Autodesk Inventor part; units mm, degrees
ref_plane "YZ Plane" through (0, 0, 0) normal (1, 0, 0) x (0, 1, 0)
ref_plane "XZ Plane" through (0, 0, 0) normal (0, 1, 0) x (-1, 0, 0)
ref_plane "XY Plane" through (0, 0, 0) normal (0, 0, 1) x (1, 0, 0)
sketch "Sketch1" plane through (0, 0, 0) normal (0, 1, 0) x (-1, 0, 0)
  line L0 (0, 0) -> (0, 5)
  line L1 (0, 5) -> (2, 5)
  line L2 (2, 5) -> (2, 3.5)
  line L3 (2, 3.5) -> (2.5, 3.5)
  line L4 (2.5, 3.5) -> (2.5, 2)
  line L5 (2.5, 2) -> (2, 2)
  line L6 (2, 2) -> (2, 1.5)
  line L7 (2, 1.5) -> (2.5, 1.5)
  line L8 (2.5, 1.5) -> (2.5, 0)
  line L9 (2.5, 0) -> (0, 0)
  dimension "d0" = 5
  dimension "d1" = 5
  dimension "d2" = 4
  dimension "d3" = 1.5
  dimension "d4" = 0.5
  dimension "d5" = 1.5
revolve "Revolution1" add sketch "Sketch1" angle 360 about axis through (0, 0, 0) along (0, 0, 1)
chamfer "Chamfer1" distance 0.5 angle 45 1 edges at (2, 0, 3.5)
hole "Hole1" at (0, 0, 0) direction (0, 0, 1) diameter 3 depth 6 tip angle 118
thread "Thread1"
properties part number "brass-insert-m3x5" material "Brass, Soft Yellow"
Work out the finished part from the listing and answer in its coordinate system (mm). A direction names the side the tool comes from. Coordinates: 2 decimals unless noted, no trailing zeros. Loops run counter-clockwise (first coordinate to the right, second up) from the corner with the lowest first, then second, coordinate; pieces in that order, holes last.
1) For a pull along Z with two mould halves and no side action, classify faces 4 (the cylindrical face through (0.54, -2.44, 0.74)), 5 (the flat face through (-2, 0, 0)), 6 (the cylindrical face through (0.434, -1.952, 1.746)) as +Z half, -Z half, draft (parallel to the pull), parting line (faces both ways), or undercut.
Results:
face 4: draft
face 5: -Z half
face 6: undercut
2) Flat-ended cylindrical pins translate along their axes: pin 1 (1 mm diameter, centred on y = 1, z = 2, fed in from -X); pin 2 (1.5 mm diameter, centred on y = 1, z = 3, fed in from -X). Find the tip coordinate at first contact, or state that the pin passes through.
Results:
pin 1: stops at x = -2.45
pin 2: stops at x = -2.49
3) Section D-D (z = 2.45) is taken. Give the vertices of the cut face in (x, y), plus the area to 3 significant figures.
Results:
outline: circle Ø5 at (0, 0); hole circle Ø3 at (0, 0)
area: 12.6 mm2
4) Consider probe 1 along Y at (x, z) = (0, 1.25); probe 2 along X at (y, z) = (0, 1.7). Determine where each line is inside the solid, lowest interval first.
Results:
probe 1: y = -2.5 to -1.5, 1.5 to 2.5
probe 2: x = -2 to -1.5, 1.5 to 2
5) For faces 1 (the flat face through (1, -2, 1.5)), 2 (the cylindrical face through (0.434, -1.952, 4.493)), 3 (the cylindrical face through (-0.07, -1.5, 2.54)), determine the directions among +Z, -Z, +X, -X, +Y, -Y from which every point of the face is accessible in a straight line to the end or side of a thin tool.
Results:
face 1: none
face 2: +Z
face 3: +Z, -Z
6) Section C-C (z = 4.7) is taken. Give the vertices of the cut face in (x, y).
Results:
outline: circle Ø4 at (0, 0); hole circle Ø3 at (0, 0)
